The listing builds one solid part. Answer for the finished solid, in the listing's coordinates (mm). A direction names the side the tool comes from. Round coordinates to 2 decimals unless told otherwise and drop trailing zeros. Order: outer loops, then holes, each group sorted by start corner. A loop starts at its lowest first (then second) coordinate and runs counter-clockwise, first axis right, second up. Notation, with made-up numbers: (11, -5) -> (25, -5) arc R13 ccw to (25, 16) -> close; hole circle Ø5 at (-31.75, -35). An arc over 180 degrees is marked (long way). Answer in a Markdown table with one row per item. Add a question column.
```python
from build123d import *

# Parameters (mm, degrees)
SKETCH1_W           = 150
SKETCH1_H           = 30
BOSS_EXTRUDE1_DEPTH = 20
SKETCH2_R           = 3
CUT_EXTRUDE1_DEPTH  = 20
SKETCH3_W           = 30
SKETCH3_H           = 10
CUT_EXTRUDE2_DEPTH  = 20
SKETCH4_W           = 30
SKETCH4_H           = 10
CUT_EXTRUDE3_DEPTH  = 20


with BuildPart() as part:
    # Sketch1 → Boss-Extrude1 (new body)
    with BuildSketch(Plane(origin=(0, 0, 0), x_dir=(1, 0, 0), z_dir=(0, 1, 0))):
        with Locations((16.197183099, 2.077464789)):
            Rectangle(SKETCH1_W, SKETCH1_H)
    extrude(amount=BOSS_EXTRUDE1_DEPTH)

    # Sketch2 → Cut-Extrude1 (cut)
    with BuildSketch(Plane(origin=(0, 20, 0), x_dir=(1, 0, 0), z_dir=(0, 1, 0))):
        with Locations(Location((-50.802816901, 2.077464789, 0), (0, 0, 270))):
            Circle(SKETCH2_R)
        with Locations(Location((83.197183099, 2.077464789, 0), (0, 0, 90))):
            Circle(SKETCH2_R)
    extrude(amount=-CUT_EXTRUDE1_DEPTH, mode=Mode.SUBTRACT)

    # Sketch3 → Cut-Extrude2 (cut)
    with BuildSketch(Plane.ZY.offset(58.802816901)):
        with Locations((-2.077464789, 10)):
            Rectangle(SKETCH3_W, SKETCH3_H)
    extrude(amount=-CUT_EXTRUDE2_DEPTH, mode=Mode.SUBTRACT)

    # Sketch4 → Cut-Extrude3 (cut)
    with BuildSketch(Plane(origin=(91.197183099, 0, 0), x_dir=(0, 0, -1), z_dir=(1, 0, 0))):
        with Locations((2.077464789, 10)):
            Rectangle(SKETCH4_W, SKETCH4_H)
    extrude(amount=-CUT_EXTRUDE3_DEPTH, mode=Mode.SUBTRACT)


solid = part.part
```
1. The part is cut by section A-A (z = -15). Give the vertices of the cut face in (x, y), then the cut area to 3 significant figures.
2. Each of these flat-tipped pins is pushed along its axis until it touches: pin 1 (6 mm diameter, centred on y = 11.5, z = 2.5, fed in from +X); pin 2 (3.5 mm diameter, centred on x = -50.8, z = -2.08, fed in from +Y); pin 3 (5 mm diameter, centred on y = 10.5, z = -1, fed in from -X). Where does it stop, or does it pass through?
3. The mould has two halves that part along X. Classify faces 1 (the flat face through (-38.803, 10, -2)), 2 (the flat face through (71.197, 10, -2)), 3 (the flat face through (15, 20, -2)), 4 (the cylindrical face through (80.223, 2.535, -1.687)): released by +X, released by -X, zero draft, split by the parting line, or undercut.
4. The part is cut by section B-B (y = 13). Give the vertices of the cut face in (x, z).
5. For faces 5 (the flat face through (15, 10, -17.077)), 6 (the flat face through (79, 15, -2)), 7 (the flat face through (-47, 5, -2)), determine the directions among +Z, -Z, +X, -X, +Y, -Y from which every point of the face is accessible in a straight line to the end or side of a thin tool.
6. Straight lines are drawn through the part: line 1 along Y through (x, z) = (-47.5, -14.25); line 2 along X through (y, z) = (18, -0.75); line 3 along X through (y, z) = (6, 1.25). For each, find the intervals that lie inside material, in ascending order.
Report:
| question | item | result |
|---|---|---|
| 1 | outline | (-58.8, 0) -> (91.2, 0) -> (91.2, 5) -> (71.2, 5) -> (71.2, 15) -> (91.2, 15) -> (91.2, 20) -> (-58.8, 20) -> (-58.8, 15) -> (-38.8, 15) -> (-38.8, 5) -> (-58.8, 5) -> close |
| 1 | area | 2,600 mm^2 |
| 2 | pin 1 | stops at x = 71.2 |
| 2 | pin 2 | passes through |
| 2 | pin 3 | stops at x = -38.8 |
| 3 | face 1 | released by -X |
| 3 | face 2 | released by +X |
| 3 | face 3 | zero draft |
| 3 | face 4 | undercut |
| 4 | outline | (-38.8, -17.08) -> (71.2, -17.08) -> (71.2, 12.92) -> (-38.8, 12.92) -> close |
| 5 | face 5 | -Z, +X, -X, +Y, -Y |
| 5 | face 6 | +Z, -Z, +X |
| 5 | face 7 | +Z, -Z, -X |
| 6 | line 1 | y = 0 to 5, 15 to 20 |
| 6 | line 2 | x = -58.8 to -53.49, -48.11 to 80.51, 85.89 to 91.2 |
| 6 | line 3 | x = -38.8 to 71.2 |
